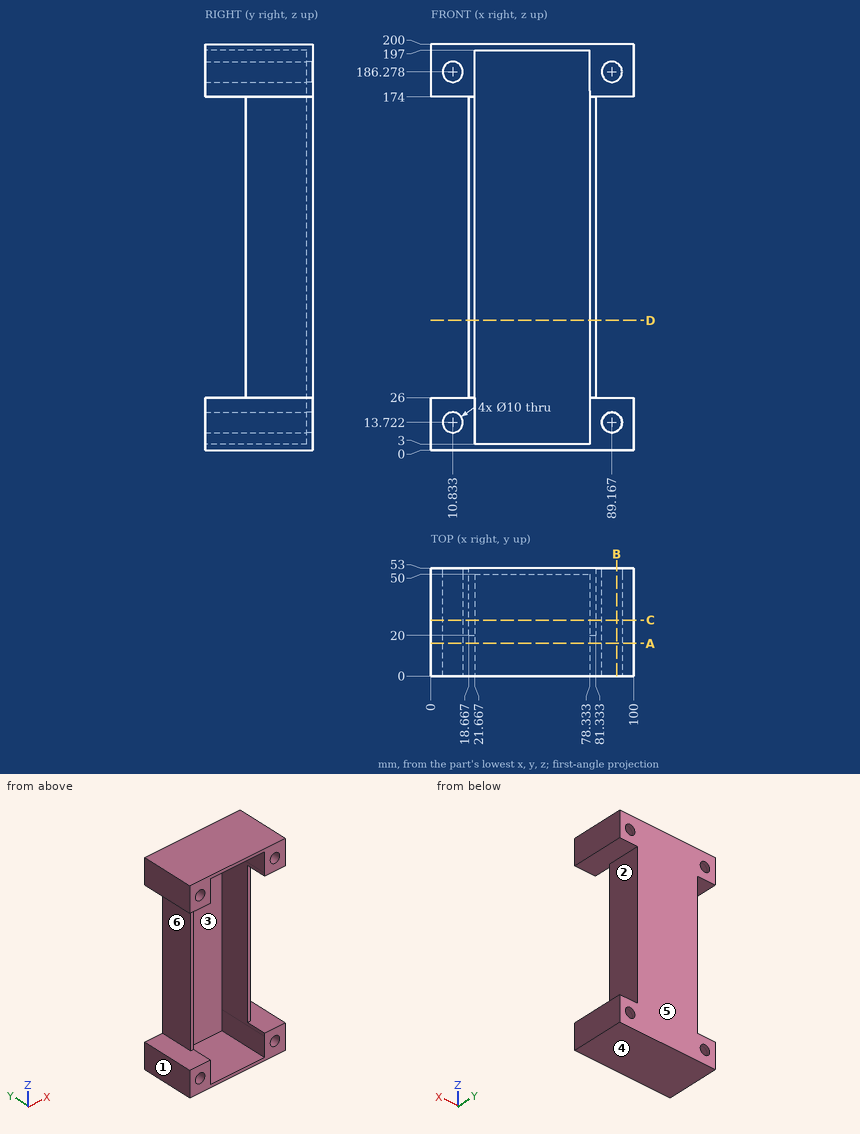
Geometry: see drawing. Coordinates: mm, zero at the bounding-box minimum. A direction names the side the tool comes from. Give positions to 0.01 mm unless a question says otherwise; leave off trailing zeros. Order: outer loops, then holes, each group sorted by start corner. A loop starts at its lowest first (then second) coordinate and runs counter-clockwise, first axis right, second up.
1. Draft query along Z for the marked faces 4, 5 and 6. Return one class per face: released by +Z, released by -Z, zero draft, split by the parting line, or undercut.
Computed:
face 4: released by -Z
face 5: zero draft
face 6: undercut
2. Cut plane B-B (x = 91.5). Return loops of the section in (y, z) (1 decimal), and give its area (3 significant figures).
Computed:
outline: (0, 0) - (53, 0) - (53, 9.3) - (0, 9.3) - close; (0, 18.1) - (53, 18.1) - (53, 26) - (0, 26) - close; (0, 174) - (53, 174) - (53, 181.9) - (0, 181.9) - close; (0, 190.7) - (53, 190.7) - (53, 200) - (0, 200) - close
area: 1,820 mm2
3. Set-up query: the marked faces 1, 2 and 3. Return all of +Z, -Z, +X, -X, +Y, -Y with unobstructed straight access to the full face (end or side cutting, diameter ignored); none if empty.
Computed:
face 1: +Z, -Z, -X, +Y, -Y
face 2: +X, +Y, -Y
face 3: -Y
4. Cut plane A-A (y = 16). Return loops of the section in (x, z).
Computed:
outline: (0, 0) - (100, 0) - (100, 26) - (78.33, 26) - (78.33, 3) - (21.67, 3) - (21.67, 26) - (0, 26) - close; (0, 174) - (21.67, 174) - (21.67, 197) - (78.33, 197) - (78.33, 174) - (100, 174) - (100, 200) - (0, 200) - close; hole circle Ø10 at (10.83, 13.72); hole circle Ø10 at (10.83, 186.28); hole circle Ø10 at (89.17, 13.72); hole circle Ø10 at (89.17, 186.28)
5. Cut plane D-D (z = 64). Return loops of the section in (x, y).
Computed:
outline: (18.67, 20) - (21.67, 20) - (21.67, 50) - (78.33, 50) - (78.33, 20) - (81.33, 20) - (81.33, 53) - (18.67, 53) - close
6. Pin query (flat end, axial travel): pin 1 Ø6.5 at (x, y) = (84, 14) entering from -Z; pin 2 Ø6 at (y, z) = (45.5, 141.5) entering from +X; pin 3 Ø9 at (x, z) = (89.17, 13.72) entering from +Y; pin 4 Ø5 at (y, z) = (44.5, 170.5) entering from -X. Return the tip coordinate at first contact, or that it passes through.
Computed:
pin 1: stops at z = 0
pin 2: stops at x = 81.33
pin 3: passes through
pin 4: stops at x = 18.67
7. Line query: probe 1 along X at (y, z) = (33.5, 174.5); probe 2 along X at (y, z) = (43, 148.5); probe 3 along Z at (x, y) = (57, 11.5). Output: solid intervals per line, ascending.
Computed:
probe 1: x = 0 to 21.67, 78.33 to 100
probe 2: x = 18.67 to 21.67, 78.33 to 81.33
probe 3: z = 0 to 3, 197 to 200
8. Cut plane C-C (y = 27.5). Return loops of the section in (x, z), and give its area (3 significant figures).
Computed:
outline: (0, 0) - (100, 0) - (100, 26) - (81.33, 26) - (81.33, 174) - (100, 174) - (100, 200) - (0, 200) - (0, 174) - (18.67, 174) - (18.67, 26) - (0, 26) - close; hole circle Ø10 at (10.83, 13.72); hole circle Ø10 at (10.83, 186.28); hole (21.67, 3) - (78.33, 3) - (78.33, 197) - (21.67, 197) - close; hole circle Ø10 at (89.17, 13.72); hole circle Ø10 at (89.17, 186.28)
area: 3,170 mm2
